from build123d import *

# Parameters (mm, degrees)
SKETCH_1_W           = 27.2
SKETCH_1_H           = 14
EXTRUDE_1_DEPTH      = 2.3
SKETCH_2_W           = 9
SKETCH_2_H           = 6.5
SKETCH_2_R           = 1.5
EXTRUDE_2_DEPTH      = 2.3
EXTRUDE_3_REACH      = 32.453
EXTRUDE_4_DEPTH      = 23.6
EXTRUDE_4_DEPTH_BACK = 23.6
SKETCH_5_R           = 1


with BuildPart() as part:
    # 草图1 → 拉伸1 (new body)
    with BuildSketch(Plane.XY):
        Rectangle(SKETCH_1_W, SKETCH_1_H)
    extrude(amount=EXTRUDE_1_DEPTH)

    # 草图2 → 拉伸2 (add)
    # profile 1 of 2: a face of its own
    with BuildSketch(Plane(origin=(0, 0, 0), x_dir=(-1, 0, 0), z_dir=(0, 0, -1))):
        with Locations((9.1, -10.25)):
            Rectangle(SKETCH_2_W, SKETCH_2_H)
        with Locations((9.1, -10.25)):
            Circle(SKETCH_2_R, mode=Mode.SUBTRACT)
    # profile 2 of 2: a face of its own
    with BuildSketch(Plane(origin=(0, 0, 0), x_dir=(-1, 0, 0), z_dir=(0, 0, -1))):
        with Locations((-9.1, 10.25)):
            Rectangle(SKETCH_2_W, SKETCH_2_H)
        with Locations((-9.1, 10.25)):
            Circle(SKETCH_2_R, mode=Mode.SUBTRACT)
    extrude(amount=-EXTRUDE_2_DEPTH)

    # 拉伸3: up to this face of the body (flat: up to its plane)
    extrude_3_end = Plane(part.part.faces().sort_by_distance((-13.6, -3.25, 1.15))[0])
    # 草图4 → 拉伸3 (add, up to the picked face)
    with BuildSketch(Plane(origin=(13.6, 0, 0), x_dir=(0, 0, -1), z_dir=(1, 0, 0)), mode=Mode.PRIVATE) as extrude_3_sk1:
        with BuildLine():
            Line((-2.3, -7), (-2.3, 7))
            ThreePointArc((-2.3, 7), (-8.509289243, 7.153612414), (-14, 4.25))
            Line((-14, 4.25), (-14, -4.25))
            ThreePointArc((-14, -4.25), (-8.509289243, -7.153612414), (-2.3, -7))
        make_face()
    extrude_3_tool1 = split(extrude(extrude_3_sk1.sketch, amount=-EXTRUDE_3_REACH, mode=Mode.PRIVATE), bisect_by=extrude_3_end, keep=Keep.BOTH, mode=Mode.PRIVATE)
    add(extrude_3_tool1.solids().sort_by(Axis((13.6, 0, 7.774162), (-1, 0, 0)))[0])

    # 草图5 → 拉伸4 (add, two sides: drawn at the far end of the back side and taken through both)
    with BuildSketch(Plane(origin=(0, 0, 0), x_dir=(0, 0, -1), z_dir=(1, 0, 0)).offset(-EXTRUDE_4_DEPTH_BACK)):
        with Locations(Location((-6.2, 0, 0), (0, 0, 270))):
            Circle(SKETCH_5_R)
    extrude(amount=EXTRUDE_4_DEPTH + EXTRUDE_4_DEPTH_BACK)


solid = part.part
Could you check a few things on this model? Use its own coordinates, in mm. A direction names the side the tool comes from. Coordinates: 2 decimals unless noted, no trailing zeros. Order: outer loops, then holes, each group sorted by start corner. A loop starts at its lowest first (then second) coordinate and runs counter-clockwise, first axis right, second up. Notation, with made-up numbers: (33.25, -19) -> (59.25, -19) arc R22 cw to (59.25, -1) -> close; hole circle Ø9 at (-31, 4). An arc over 180 degrees is marked (long way). One line per question, with ' | ' between items.
Q1. On a 3-axis mill with a long thin cutter (end or side, diameter ignored), from which of +Z, -Z, +X, -X, +Y, -Y can I reach the whole of each face in a straight line? I mean faces 1 (the face through (-8, -9, 2.3)), 2 (the face through (4, -7, 1)), 3 (the face through (10, 12, 2.3)), 4 (the face through (-18.67, 0.13, 5.21)). Say none if no direction works.
Return value:
face 1: +X, -X, -Y | face 2: -Z, +X, -Y | face 3: +X, -X, +Y | face 4: -X
Q2. Imagine slicing it at D-D on y = 0. Please give me the cut outline in (x, z).
Return value:
outline: (-23.6, 5.2) -> (-13.6, 5.2) -> (-13.6, 0) -> (13.6, 0) -> (13.6, 5.2) -> (23.6, 5.2) -> (23.6, 7.2) -> (13.6, 7.2) -> (13.6, 14) -> (-13.6, 14) -> (-13.6, 7.2) -> (-23.6, 7.2) -> close
Q3. I'm going to push flat-ended pins straight in: P1, Ø1.8, axis at x = -9.1, y = -10.25, coming from the +Z side; P2, Ø3, axis at x = -4, y = -6, coming from the +Z side; P3, Ø1.2, axis at y = -11, z = 1.5, coming from the +X side; P4, Ø3, axis at x = 15, z = 4, coming from the -Y side. Where does each tip first touch, or does it pass through?
Return value:
P1: through | P2: z = 13.72 | P3: x = -4.6 | P4: y = -7.42
Q4. Imagine slicing it at C-C on z = 1. Please give me the cut outline in (x, y), and give its area (3 significant figures).
Return value:
outline: (-13.6, -13.5) -> (-4.6, -13.5) -> (-4.6, -7) -> (13.6, -7) -> (13.6, 13.5) -> (4.6, 13.5) -> (4.6, 7) -> (-13.6, 7) -> close; hole circle Ø3 at (-9.1, -10.25); hole circle Ø3 at (9.1, 10.25) | area: 484 mm²
Q5. If I drill on L1, parallel to Y at x = -9.1, z = 1.4; L2, parallel to Y at x = 9.1, z = 1.2; L3, parallel to X at y = 3.5, z = 2.25, over which ranges is the centre line in solid material (lowest first)?
Return value:
L1: -13.5 to -11.75, -8.75 to 7 | L2: -7 to 8.75, 11.75 to 13.5 | L3: -13.6 to 13.6
Q6. Thinking about a two-plate mould opening in Y: for faces 5 (the face through (10.6, 10.3, 1.1)), 6 (the face through (18.53, 0.13, 5.21)), 7 (the face through (-4.6, -10, 1)), 8 (the face through (-5, 7, 1)), which applies, pulls with the +Y half, pulls with the -Y half, needs draft (parallel to the pull), parting line crosses it, or undercut?
Return value:
face 5: undercut | face 6: parting line crosses it | face 7: needs draft | face 8: pulls with the +Y half
Q7. Imagine slicing it at A-A on x = 9.1. Please give me the cut outline in (y, z).
Return value:
outline: (-7, 0) -> (8.75, 0) -> (8.75, 2.3) -> (7, 2.3) arc R12.28 ccw to (4.25, 14) -> (-4.25, 14) arc R12.28 ccw to (-7, 2.3) -> close; (11.75, 0) -> (13.5, 0) -> (13.5, 2.3) -> (11.75, 2.3) -> close
Q8. Imagine slicing it at B-B on y = -10.25. Please give me the cut outline in (x, z), and give its area (3 significant figures).
Return value:
outline: (-13.6, 0) -> (-10.6, 0) -> (-10.6, 2.3) -> (-13.6, 2.3) -> close; (-7.6, 0) -> (-4.6, 0) -> (-4.6, 2.3) -> (-7.6, 2.3) -> close | area: 13.8 mm²
